Autodesk Inventor part; units mm, degrees
sketch "Skizze1" plane through (0, 0, 0) normal (0, 0, 1) x (1, 0, 0)
  line L0 (-100, 80) -> (100, 80)
  line L1 (100, 80) -> (100, -80)
  line L2 (100, -80) -> (-100, -80)
  line L3 (-100, -80) -> (-100, 80)
  line L4 (0, -112) -> (0, 112)
  line L5 (-140, 0) -> (140, 0)
  point P0 (0, 0)
  dimension "d0" = 160
  dimension "d1" = 200
extrude "Extrusion1" add sketch "Skizze1" along normal blind 100
sketch "Skizze2" plane through (0, 0, 100) normal (0, 0, 1) x (1, 0, 0)
  line L0 (-95, 75) -> (95, 75)
  line L1 (95, 75) -> (95, -75)
  line L2 (95, -75) -> (-95, -75)
  line L3 (-95, -75) -> (-95, 75)
  line L4 (0, -112) -> (0, 112)
  line L5 (-140, 0) -> (140, 0)
  point P0 (0, 0)
  dimension "d4" = 150
  dimension "d5" = 190
extrude "Extrusion2" cut sketch "Skizze2" against normal blind 95
sketch "Skizze3" plane through (0, 0, 5) normal (0, 0, 1) x (1, 0, 0)
  line L0 (100, -80) -> (100, 80)
  line L1 (100, -80) -> (125, -80)
  line L2 (125, -80) -> (125, 80)
  line L3 (125, 80) -> (100, 80)
  line L4 (100, 80) -> (100, -80)
  point P0 (0, 0)
extrude "Extrusion3" add sketch "Skizze3" against normal blind 5
sketch "Skizze4" plane through (0, 0, 5) normal (0, 0, 1) x (1, 0, 0)
  point P0 (0, 0)
sketch "Skizze5" plane through (0, 0, 5) normal (0, 0, 1) x (1, 0, 0)
  line L0 (100, -80) -> (100, 80)
  line L1 (100, -80) -> (125, -80)
  line L2 (125, -80) -> (125, 80)
  line L3 (125, 80) -> (100, 80)
  point P0 (0, 0)
  point P1 (112.5, 55)
  point P2 (112.5, -55)
hole "Bohrung2" at (112.5, 55, 5) at (112.5, -55, 5) direction (0, 0, -1) diameter 6.4 depth 8 tip angle 118
mirror "Spiegeln1" about plane through (0, 0, 0) normal (1, 0, 0) of "Extrusion3", "Bohrung2"
fillet "Rundung1" radius 2 10 edges at (125, 0, 5) (-125, 0, 5) (-112.5, -80, 5) (-100, -80, 52.5) (112.5, -80, 5) (100, -80, 52.5) (112.5, 80, 5) (-112.5, 80, 5) (-100, 80, 52.5) (100, 80, 52.5)
properties part number "Box"
The listing builds one solid part. Answer for the finished solid, in the listing's coordinates (mm). A direction names the side the tool comes from. Round coordinates to 2 decimals unless told otherwise and drop trailing zeros. Order: outer loops, then holes, each group sorted by start corner. A loop starts at its lowest first (then second) coordinate and runs counter-clockwise, first axis right, second up. Notation, with made-up numbers: (-31.75, -7) -> (23.25, -7) arc R10 cw to (23.25, 4) -> close; hole circle Ø11 at (4, 4). An arc over 180 degrees is marked (long way). One line per item, written item: value.
Item 1: Find section B-B, the plane x = 112.5. Give the vertices of the cut face in (y, z).
Taken from the geometry:
outline: (-80, 0) -> (-58.2, 0) -> (-58.2, 5) -> (-78, 5) arc R2 ccw to (-80, 3) -> close; (-51.8, 0) -> (51.8, 0) -> (51.8, 5) -> (-51.8, 5) -> close; (58.2, 0) -> (80, 0) -> (80, 3) arc R2 ccw to (78, 5) -> (58.2, 5) -> close
Item 2: Find section A-A, the plane z = 25. Give the vertices of the cut face in (x, y).
Taken from the geometry:
outline: (-100, -78) arc R2 ccw to (-98, -80) -> (98, -80) arc R2 ccw to (100, -78) -> (100, 78) arc R2 ccw to (98, 80) -> (-98, 80) arc R2 ccw to (-100, 78) -> close; hole (-95, -75) -> (95, -75) -> (95, 75) -> (-95, 75) -> close
Item 3: Find section C-C, the plane y = 55. Give the vertices of the cut face in (x, z).
Taken from the geometry:
outline: (-125, 0) -> (-115.7, 0) -> (-115.7, 5) -> (-123, 5) arc R2 ccw to (-125, 3) -> close; (-109.3, 0) -> (109.3, 0) -> (109.3, 5) -> (100, 5) -> (100, 100) -> (95, 100) -> (95, 5) -> (-95, 5) -> (-95, 100) -> (-100, 100) -> (-100, 5) -> (-109.3, 5) -> close; (115.7, 0) -> (125, 0) -> (125, 3) arc R2 ccw to (123, 5) -> (115.7, 5) -> close
Item 4: Straight lines are drawn through the part: L1, parallel to Y at x = -112.5, z = 3.3; L2, parallel to X at y = -55, z = 2; L3, parallel to Y at x = 74, z = 33.5. For each, find the intervals that lie inside material, in ascending order.
Taken from the geometry:
L1: y = -79.98 to -58.2, -51.8 to 51.8, 58.2 to 79.98
L2: x = -125 to -115.7, -109.3 to 109.3, 115.7 to 125
L3: y = -80 to -75, 75 to 80
Item 5: For a pull along X with two mould halves and no side action, classify faces 4 (the cylindrical face through (-112.6, 58.2, 2.5)), 5 (the flat face through (-2, 1, 0)), 6 (the cylindrical face through (112.4, 58.2, 2.5)), 7 (the flat face through (-100, -1, 52)) as released by +X, released by -X, zero draft, split by the parting line, or undercut.
Taken from the geometry:
face 4: undercut
face 5: zero draft
face 6: undercut
face 7: released by -X
Item 6: Given P1, Ø1, axis at y = -35.5, z = 63, coming from the +X side; P2, Ø11.5, axis at x = -113, y = -32, coming from the +Z side; P3, Ø12, axis at y = -53, z = 64.5, coming from the -X side, each flat-ended and moving along its own axis, determine where each tip first touches the part or whether it passes through.
Taken from the geometry:
P1: stops at x = 100
P2: stops at z = 5
P3: stops at x = -100
Item 7: For faces 1 (the flat face through (95, 1, 53)), 2 (the flat face through (-112, 1, 5)), 3 (the flat face through (111, 1, 5)), determine the directions among +Z, -Z, +X, -X, +Y, -Y from which every point of the face is accessible in a straight line to the end or side of a thin tool.
Taken from the geometry:
face 1: +Z
face 2: +Z, -X, +Y, -Y
face 3: +Z, +X, +Y, -Y
Item 8: Find section D-D, the plane x = -33.5. Give the vertices of the cut face in (y, z), then the cut area to 3 significant figures.
Taken from the geometry:
outline: (-80, 0) -> (80, 0) -> (80, 100) -> (75, 100) -> (75, 5) -> (-75, 5) -> (-75, 100) -> (-80, 100) -> close
area: 1,750 mm2
